Input: part model. Units: mm. Frame: model coordinates. Round coordinates to 2 decimals unless told otherwise and drop trailing zeros. Loops run counter-clockwise (first coordinate to the right, second up) from the corner with the lowest first, then second, coordinate; pieces in that order, holes last. Notation, with made-up numbers: M 6,72.5 L 62,72.5 A19 ccw 62,95.5 Z; hole C -14.5,42 d8. An arc over 180 degrees is marked long. Use one line per item in the form item = value. Start each with the question number.
Q1. Ray query, line 1 along Y through (x, z) = (31.5, 0.25); line 2 along X through (y, z) = (-1.5, 2.2); line 3 along X through (y, z) = (1.25, 0.65). Return the intervals inside material, ascending.
Q2. Section query B-B, the plane x = 56. Output: boundary loops of the cut face in (y, z), and give its area (3 significant figures).
Q3. Section query C-C, the plane y = -1.75. Output: boundary loops of the cut face in (x, z), and give its area (3 significant figures).
Q4. First-contact query: P1, Ø0.8, axis at x = -0.5, z = 2, coming from the -Y side; P2, Ø1.3, axis at x = 0, z = 1, coming from the +Y side. Flat tips, straight axial feed; report the tip coordinate or a pass-through.
Q5. Section query A-A, the plane z = 1.25. Output: boundary loops of the cut face in (x, y).
```python
from build123d import *

# Parameters (mm, degrees)
BOSS_EXTRUDE1_DEPTH = 2.54
SKETCH3_W           = 69.160945518
SKETCH3_H           = 10.6172
BOSS_EXTRUDE2_DEPTH = 2.54


with BuildPart() as part:
    # Sketch1 → Boss-Extrude1 (new body)
    with BuildSketch(Plane.XY):
        Polygon((70.693406338, 2.6543), (72.680472759, 6.096), (78.253057557, 6.096), (78.253057557, 3.556), (74.146942443, 3.556), (72.093884886, 0), (74.146942443, -3.556), (78.253057557, -3.556), (78.253057557, -6.096), (72.680472759, -6.096), (70.693406338, -2.6543), (4.597382459, -2.6543), (3.064921639, -5.3086), (-1.598451955, -5.3086), (-1.598451955, -2.7686), (1.598451955, -2.7686), (3.196903911, 0), (1.598451955, 2.7686), (-1.598451955, 2.7686), (-1.598451955, 5.3086), (3.064921639, 5.3086), (4.597382459, 2.6543), align=None)
    extrude(amount=BOSS_EXTRUDE1_DEPTH)

    # Sketch3 → Boss-Extrude2 (add)
    with BuildSketch(Plane.XY.offset(2.54)):
        with Locations((37.645394398, 0)):
            Rectangle(SKETCH3_W, SKETCH3_H)
    extrude(amount=-BOSS_EXTRUDE2_DEPTH)


solid = part.part
```
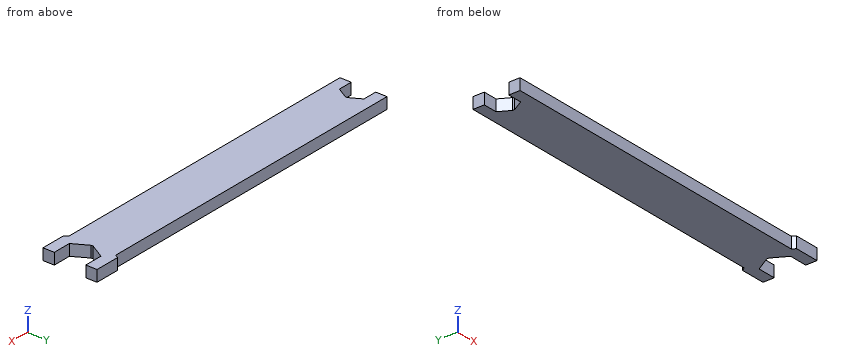
Results found:
q1.line_1 = -5.31 to 5.31
q1.line_2 = 2.33 to 72.96
q1.line_3 = 2.48 to 72.82
q2.outline = M -5.31,0 L 5.31,0 L 5.31,2.54 L -5.31,2.54 Z
q2.area = 27.0 mm²
q3.outline = M 2.19,0 L 73.1,0 L 73.1,2.54 L 2.19,2.54 Z
q3.area = 180 mm²
q4.P1 = -5.31
q4.P2 = 5.31
q5.outline = M -1.6,-5.31 L 72.23,-5.31 L 72.68,-6.1 L 78.25,-6.1 L 78.25,-3.56 L 74.15,-3.56 L 72.23,-0.23 L 72.23,0.23 L 74.15,3.56 L 78.25,3.56 L 78.25,6.1 L 72.68,6.1 L 72.23,5.31 L -1.6,5.31 L -1.6,2.77 L 1.6,2.77 L 3.06,0.23 L 3.06,-0.23 L 1.6,-2.77 L -1.6,-2.77 Z
